```python
from build123d import *

# Parameters (mm, degrees)
SKETCH1_W           = 190
SKETCH1_H           = 70
BOSS_EXTRUDE1_DEPTH = 3
FILLET6_R           = 2.54
FILLET7_R           = 2.54
SKETCH2_R           = 12.5
CUT_EXTRUDE1_DEPTH  = 6.578222623


with BuildPart() as part:
    # Sketch1 → Boss-Extrude1 (new body)
    with BuildSketch(Plane(origin=(0, 0, 0), x_dir=(1, 0, 0), z_dir=(0, 1, 0))):
        Rectangle(SKETCH1_W, SKETCH1_H)
    extrude(amount=BOSS_EXTRUDE1_DEPTH)

    # Fillet6
    fillet6_edges = [part.edges().sort_by_distance(p)[0] for p in [
        (95, 1.5, 35),
        (-95, 1.5, 35),
        (-95, 1.5, -35),
        (95, 1.5, -35),
    ]]
    fillet(fillet6_edges, radius=FILLET6_R)

    # Fillet7
    fillet7_edges = [part.edges().sort_by_distance(p)[0] for p in [
        (0, 3, -35),
        (95, 3, 0),
        (-95, 3, 0),
        (0, 3, 35),
        (-94.256051224, 3, -34.256051224),
        (-94.256051224, 3, 34.256051224),
        (94.256051224, 3, 34.256051224),
        (94.256051224, 3, -34.256051224),
    ]]
    fillet(fillet7_edges, radius=FILLET7_R)

    # Sketch2 → Cut-Extrude1 (cut)
    with BuildSketch(Plane(origin=(0, 3, 0), x_dir=(1, 0, 0), z_dir=(0, 1, 0))):
        with BuildLine():
            ThreePointArc((-74.901262656, 4.383937879), (-75, 2.982154077), (-74.901262656, 1.580370275))
            Line((-74.901262656, 1.580370275), (-71.372168947, 1.580370275))
            Line((-71.372168947, 1.580370275), (-71.372168947, 4.383937879))
            Line((-71.372168947, 4.383937879), (-74.901262656, 4.383937879))
        make_face()
        with BuildLine():
            Line((-71.372168947, 1.580370275), (-74.901262656, 1.580370275))
            ThreePointArc((-74.901262656, 1.580370275), (-64.297371562, -6.993131046), (-55, 2.982154077))
            ThreePointArc((-55, 2.982154077), (-64.297371562, 12.9574392), (-74.901262656, 4.383937879))
            Line((-74.901262656, 4.383937879), (-71.372168947, 4.383937879))
            Line((-71.372168947, 4.383937879), (-71.372168947, 1.580370275))
        make_face()
        with Locations(Location((-28.415448, 2.982154077, 0), (0, 0, 270))):
            Circle(SKETCH2_R)
        with BuildLine():
            Line((-78.627831053, 4.383937879), (-78.627831053, 1.580370275))
            Line((-78.627831053, 1.580370275), (-74.901262656, 1.580370275))
            ThreePointArc((-74.901262656, 1.580370275), (-75, 2.982154077), (-74.901262656, 4.383937879))
            Line((-74.901262656, 4.383937879), (-78.627831053, 4.383937879))
        make_face()
    extrude(amount=-CUT_EXTRUDE1_DEPTH, mode=Mode.SUBTRACT)


solid = part.part
```
The model under review builds one solid part; all positions refer to its coordinate system, in mm. Give positions to 0.01 mm unless a question says otherwise; leave off trailing zeros. Write each loop counter-clockwise with the first axis right and the second up, starting at its lowest first coordinate (ties: lowest second). Pieces come first, ordered by that corner, then holes.
(1) For P1, Ø12, axis at x = -61.5, z = -4, coming from the -Y side; P2, Ø0.8, axis at y = 1, z = -3.5, coming from the +X side; P3, Ø1.5, axis at x = 67.5, y = 2, coming from the -Z side; P4, Ø0.9, axis at x = -77, y = 2, coming from the +Z side, all flat-tipped, find the tip position at first contact; note any pin that passes through.
(2) Consider section B-B, the plane z = 1.5. Give the boundary of the cut face in (x, y), and give its area (3 significant figures).
(3) To check wall thickness, follow L1, parallel to X at y = 1.2, z = -5.5; L2, parallel to Z at x = -29, y = 0.5; L3, parallel to X at y = 2.3, z = -7. State the ranges of each line that lie inside material, in increasing order.
(4) Consider section D-D, the plane x = -39. Give the boundary of the cut face in (y, z).
(5) Consider section C-C, the plane y = 2.4. Give the boundary of the cut face in (x, z).
(6) The part is to be moulded in two halves that separate along Z. For faces 1 (the cylindrical face through (-16.02, 1.52, -4.61)), 2 (the flat face through (-1, 3, 0)), say which applies: released by +Z, released by -Z, zero draft, split by the parting line, or undercut.
(7) Consider section A-A, the plane x = -65. Give the boundary of the cut face in (y, z).
Returned:
1. P1: passes through
1. P2: stops at x = 95
1. P3: stops at z = -34.87
1. P4: stops at z = 34.75
2. outline: (-95, 0) - (-73.94, 0) - (-73.94, 3) - (-92.46, 3) arc R2.54 ccw to (-95, 0.46) - close; (-56.06, 0) - (-40.08, 0) - (-40.08, 3) - (-56.06, 3) - close; (-16.75, 0) - (95, 0) - (95, 0.46) arc R2.54 ccw to (92.46, 3) - (-16.75, 3) - close
2. area: 444 mm2
3. L1: x = -94.89 to -74.68, -55.32 to -40.66, -16.17 to 94.89
3. L2: z = -35 to -15.47, 9.5 to 35
3. L3: x = -94.21 to -74.16, -55.84 to -40.25, -16.58 to 94.21
4. outline: (0, -35) - (0.46, -35) arc R2.54 ccw to (3, -32.46) - (3, -9.63) - (0, -9.63) - close; (0, 3.67) - (3, 3.67) - (3, 32.46) arc R2.54 ccw to (0.46, 35) - (0, 35) - close
5. outline: (-94.1, -32.46) arc R1.64 ccw to (-92.46, -34.1) - (92.46, -34.1) arc R1.64 ccw to (94.1, -32.46) - (94.1, 32.46) arc R1.64 ccw to (92.46, 34.1) - (-92.46, 34.1) arc R1.64 ccw to (-94.1, 32.46) - close; hole (-78.63, -4.38) - (-74.9, -4.38) arc R10 ccw (long way) to (-74.9, -1.58) - (-78.63, -1.58) - close; hole circle Ø25 at (-28.42, -2.98)
6. face 1: undercut
6. face 2: zero draft
7. outline: (0, -35) - (0.46, -35) arc R2.54 ccw to (3, -32.46) - (3, -12.98) - (0, -12.98) - close; (0, 7.02) - (3, 7.02) - (3, 32.46) arc R2.54 ccw to (0.46, 35) - (0, 35) - close
